from build123d import *

# Parameters (mm, degrees)
F1_DEPTH = 1
F3_DEPTH = 2
F4_DEPTH = 25


# Not quite as in the source:
# - a feature names something its author has since deleted; it is built from what else it names


with BuildPart() as f1:
    # F0 (on Top) → F1 (new body)
    with BuildSketch(Plane.XY):
        with BuildLine():
            ThreePointArc((-10.9, 13.9), (-13.0213203436, 13.0213203436), (-13.9, 10.9))
            Line((-13.9, 10.9), (-13.9, -10.9))
            ThreePointArc((-13.9, -10.9), (-13.0213203436, -13.0213203436), (-10.9, -13.9))
            Line((-10.9, -13.9), (10.9, -13.9))
            ThreePointArc((10.9, -13.9), (13.0213203436, -13.0213203436), (13.9, -10.9))
            Line((13.9, -10.9), (13.9, 10.9))
            ThreePointArc((13.9, 10.9), (13.0213203436, 13.0213203436), (10.9, 13.9))
            Line((10.9, 13.9), (-10.9, 13.9))
        make_face()
    extrude(amount=F1_DEPTH)

    # F2 (on face) → F3 (join)
    with BuildSketch(Plane.XY.offset(1)):
        Polygon((-0.8220698815, 9.9003828379), (-0.9031134541, 9.8906987285), (-2.8628115953, 9.6565292491), (-1.3706095432, 8.3073079855), (-1.7693148693, 6.2910923774), (-0.9031134541, 6.7887921262), (-0.0250134015, 7.2933285631), (0.9031134541, 6.7749159991), (1.7693148693, 6.2910923774), (1.3551504109, 8.2597296685), (2.8628115953, 9.6565292491), (0.9031134541, 9.8666282056), (0.8625424153, 9.8709778209), (0, 11.7364836228), align=None)
        Polygon((-1.1949065374, 2.0178125706), (-2.11299252, 0.8704443462), (2.11299252, 0.8704443462), (1.1949065374, 2.0178125706), (2.3687703069, 2.0178125706), (0.9031134541, 4.6618687775), (0, 6.2910923774), (-0.9324762655, 4.6088980406), (-2.3687703069, 2.0178125706), align=None)
        Polygon((3.5059938878, -0.8704443462), (-3.5059938878, -0.8704443462), (-5.8554494827, -3.8066515699), (-3.1518915202, -3.8066515699), (-9.0449256822, -9.6830716357), (-1.1949065374, -9.6830716357), (-1.1949065374, -11.6795562208), (0, -11.6795562208), (1.1949065374, -11.6795562208), (1.1949065374, -9.6830716357), (9.0449256822, -9.6830716357), (3.1518915202, -3.8066515699), (5.8554494827, -3.8066515699), align=None)
        Polygon((2.11299252, 0.8704443462), (-2.11299252, 0.8704443462), (-3.5059938878, -0.8704443462), (3.5059938878, -0.8704443462), align=None)
    extrude(amount=F3_DEPTH)

    # F2 (on face) → F4 (cut)
    with BuildSketch(Plane.XY.offset(1)):
        with BuildLine():
            ThreePointArc((-10.9, 13.4), (-12.667766953, 12.667766953), (-13.4, 10.9))
            Line((-13.4, 10.9), (-13.4, 0.8704443462))
            Line((-13.4, 0.8704443462), (-2.11299252, 0.8704443462))
            Line((-2.11299252, 0.8704443462), (-1.1949065374, 2.0178125706))
            Line((-1.1949065374, 2.0178125706), (-2.3687703069, 2.0178125706))
            Line((-2.3687703069, 2.0178125706), (-0.9324762655, 4.6088980406))
            Line((-0.9324762655, 4.6088980406), (-0.9031134541, 6.2910923774))
            Line((-0.9031134541, 6.2910923774), (-0.9031134541, 6.7887921262))
            Line((-0.9031134541, 6.7887921262), (-1.7693148693, 6.2910923774))
            Line((-1.7693148693, 6.2910923774), (-1.3706095432, 8.3073079855))
            Line((-1.3706095432, 8.3073079855), (-2.8628115953, 9.6565292491))
            Line((-2.8628115953, 9.6565292491), (-0.9031134541, 9.8906987285))
            Line((-0.9031134541, 9.8906987285), (-0.9031134541, 13.4))
            Line((-0.9031134541, 13.4), (-10.9, 13.4))
        make_face()
        with BuildLine():
            Line((1.1949065374, 2.0178125706), (2.11299252, 0.8704443462))
            Line((2.11299252, 0.8704443462), (13.4, 0.8704443462))
            Line((13.4, 0.8704443462), (13.4, 10.9))
            ThreePointArc((13.4, 10.9), (12.667766953, 12.667766953), (10.9, 13.4))
            Line((10.9, 13.4), (0.9031134541, 13.4))
            Line((0.9031134541, 13.4), (0.9031134541, 9.8666282056))
            Line((0.9031134541, 9.8666282056), (2.8628115953, 9.6565292491))
            Line((2.8628115953, 9.6565292491), (1.3551504109, 8.2597296685))
            Line((1.3551504109, 8.2597296685), (1.7693148693, 6.2910923774))
            Line((1.7693148693, 6.2910923774), (0.9031134541, 6.7749159991))
            Line((0.9031134541, 6.7749159991), (0.9031134541, 6.2910923774))
            Line((0.9031134541, 6.2910923774), (0.9031134541, 4.6618687775))
            Line((0.9031134541, 4.6618687775), (2.3687703069, 2.0178125706))
            Line((2.3687703069, 2.0178125706), (1.1949065374, 2.0178125706))
        make_face()
        with BuildLine():
            Line((-3.5059938878, -0.8704443462), (-13.4, -0.8704443462))
            Line((-13.4, -0.8704443462), (-13.4, -10.9))
            ThreePointArc((-13.4, -10.9), (-12.667766953, -12.667766953), (-10.9, -13.4))
            Line((-10.9, -13.4), (-1.1949065374, -13.4))
            Line((-1.1949065374, -13.4), (-1.1949065374, -11.6795562208))
            Line((-1.1949065374, -11.6795562208), (-1.1949065374, -9.6830716357))
            Line((-1.1949065374, -9.6830716357), (-9.0449256822, -9.6830716357))
            Line((-9.0449256822, -9.6830716357), (-3.1518915202, -3.8066515699))
            Line((-3.1518915202, -3.8066515699), (-5.8554494827, -3.8066515699))
            Line((-5.8554494827, -3.8066515699), (-3.5059938878, -0.8704443462))
        make_face()
        with BuildLine():
            Line((13.4, -0.8704443462), (3.5059938878, -0.8704443462))
            Line((3.5059938878, -0.8704443462), (5.8554494827, -3.8066515699))
            Line((5.8554494827, -3.8066515699), (3.1518915202, -3.8066515699))
            Line((3.1518915202, -3.8066515699), (9.0449256822, -9.6830716357))
            Line((9.0449256822, -9.6830716357), (1.1949065374, -9.6830716357))
            Line((1.1949065374, -9.6830716357), (1.1949065374, -11.6795562208))
            Line((1.1949065374, -11.6795562208), (1.1949065374, -13.4))
            Line((1.1949065374, -13.4), (10.9, -13.4))
            ThreePointArc((10.9, -13.4), (12.667766953, -12.667766953), (13.4, -10.9))
            Line((13.4, -10.9), (13.4, -0.8704443462))
        make_face()
    extrude(amount=-F4_DEPTH, mode=Mode.SUBTRACT)


solid = f1.part
Part model, mm, in its own coordinate system. A direction names the side the tool comes from. Round coordinates to 2 decimals unless told otherwise and drop trailing zeros. Loops run counter-clockwise (first coordinate to the right, second up) from the corner with the lowest first, then second, coordinate; pieces in that order, holes last. Notation, with made-up numbers: (70.25, 64.25) - (110.25, 64.25) arc R12 ccw to (110.25, 68.25) - close; hole circle Ø9 at (19, 11.25). An arc over 180 degrees is marked (long way). Answer as a JSON object with one key per item and string values.
Item 1: Band-saw the part on D-D on z = 0.6. State how many separate pieces and enclosed holes the cut face has, plus the area to 3 significant figures.
Output:
{"separate pieces": "1", "enclosed holes": "4", "area": "241 mm2"}
Item 2: Band-saw the part on B-B on x = 7.25. List the corners of the cut face in (y, z).
Output:
{"outline": "(-13.9, 0) - (-13.4, 0) - (-13.4, 1) - (-13.9, 1) - close; (-9.68, 0) - (-7.89, 0) - (-7.89, 3) - (-9.68, 3) - close; (-0.87, 0) - (0.87, 0) - (0.87, 1) - (-0.87, 1) - close; (13.4, 0) - (13.9, 0) - (13.9, 1) - (13.4, 1) - close"}
Item 3: Pin check, flat tips, straight feed: pin 1 (5 mm diameter, centred on x = 7, y = 5.5, fed in from -Z); pin 2 (0.6 mm diameter, centred on x = 0, z = 2, fed in from -Y). Stop position of each tip, or through.
Output:
{"pin 1": "through", "pin 2": "y = -11.68"}
Item 4: Band-saw the part on A-A on y = -6.5. List the corners of the cut face in (x, z), plus the area to 3 significant figures.
Output:
{"outline": "(-13.9, 0) - (-13.4, 0) - (-13.4, 1) - (-13.9, 1) - close; (-5.85, 0) - (5.85, 0) - (5.85, 3) - (-5.85, 3) - close; (13.4, 0) - (13.9, 0) - (13.9, 1) - (13.4, 1) - close", "area": "36.1 mm2"}
Item 5: Band-saw the part on C-C on y = 3.25. List the corners of the cut face in (x, z).
Output:
{"outline": "(-13.9, 0) - (-13.4, 0) - (-13.4, 1) - (-13.9, 1) - close; (-1.69, 0) - (1.69, 0) - (1.69, 3) - (-1.69, 3) - close; (13.4, 0) - (13.9, 0) - (13.9, 1) - (13.4, 1) - close"}
Item 6: Tool access for faces 1 (the face through (-1, -1, 0)), 2 (the face through (1.56, 7.29, 1.52)): list every direction of +Z, -Z, +X, -X, +Y, -Y with a clear straight run to the whole face (end or side of a thin tool).
Output:
{"face 1": "-Z, +X, -X, +Y, -Y", "face 2": "+Z, -Z"}
Item 7: Wall check: L1, parallel to X at y = 11, z = 0.9; L2, parallel to X at y = -11.5, z = 0.6; L3, parallel to Y at x = 3.5, z = 2.35. Give the ranges that are in metal, low to high.
Output:
{"L1": "-13.9 to -13.4, -0.9 to 0.9, 13.4 to 13.9", "L2": "-13.84 to -13.33, -1.19 to 1.19, 13.33 to 13.84", "L3": "-9.68 to -4.15, -3.81 to -0.86"}
Item 8: Pull direction X, two halves, no side cores. Call faces 3 (the face through (-3.2, 0.1, 1)), 4 (the face through (12.648, -12.687, 0.507)): pulls with the +X half, pulls with the -X half, needs draft (parallel to the pull), parting line crosses it, or undercut.
Output:
{"face 3": "needs draft", "face 4": "undercut"}
